Geometry: final body of the model. Coordinates: model frame, mm. A direction names the side the tool comes from. Coordinates: 2 decimals unless noted, no trailing zeros. Order: outer loops, then holes, each group sorted by start corner. A loop starts at its lowest first (then second) coordinate and runs counter-clockwise, first axis right, second up. Notation, with made-up numbers: (32.5, 34.5) -> (63.5, 34.5) arc R21 cw to (63.5, 46.5) -> close; hole circle Ø4 at (2, 67.5). An arc over 180 degrees is marked (long way). Use CSV: the item, a comma, the result in double quotes. Start each with the question number.
from build123d import *

# Parameters (mm, degrees)
SKETCH_R    = 7.65
SKETCH_R_2  = 1.6
PAD_DEPTH   = 5
FILLET_R    = 5
FILLET001_R = 5
FILLET002_R = 5


with BuildPart() as part:
    # Sketch → Pad (new body)
    with BuildSketch(Plane.XY):
        Polygon((66, 12.5), (66, -12.5), (41, -12.5), (37, -8.5), (-37, -8.5), (-41, -12.5), (-66, -12.5), (-66, 12.5), (-41, 12.5), (-37, 8.5), (37, 8.5), (41, 12.5), align=None)
        with Locations((54, 0)):
            Circle(SKETCH_R, mode=Mode.SUBTRACT)
        with Locations((45.5, 8.5)):
            Circle(SKETCH_R_2, mode=Mode.SUBTRACT)
        with Locations((62.5, 8.5)):
            Circle(SKETCH_R_2, mode=Mode.SUBTRACT)
        with Locations((62.5, -8.5)):
            Circle(SKETCH_R_2, mode=Mode.SUBTRACT)
        with Locations((45.5, -8.5)):
            Circle(SKETCH_R_2, mode=Mode.SUBTRACT)
        with Locations((-54, 0)):
            Circle(SKETCH_R, mode=Mode.SUBTRACT)
        with Locations((-45.5, 8.5)):
            Circle(SKETCH_R_2, mode=Mode.SUBTRACT)
        with Locations((-62.5, 8.5)):
            Circle(SKETCH_R_2, mode=Mode.SUBTRACT)
        with Locations((-62.5, -8.5)):
            Circle(SKETCH_R_2, mode=Mode.SUBTRACT)
        with Locations((-45.5, -8.5)):
            Circle(SKETCH_R_2, mode=Mode.SUBTRACT)
        with BuildLine():
            ThreePointArc((-28, 5), (-33, 0), (-28, -5))
            Line((-11.5, -5), (-28, -5))
            ThreePointArc((-11.5, -5), (-6.5, 0), (-11.5, 5))
            Line((-28, 5), (-11.5, 5))
        make_face(mode=Mode.SUBTRACT)
        with BuildLine():
            ThreePointArc((18, -5), (23, 0), (18, 5))
            Line((18, 5), (12, 5))
            ThreePointArc((12, 5), (7, 0), (12, -5))
            Line((18, -5), (12, -5))
        make_face(mode=Mode.SUBTRACT)
    extrude(amount=PAD_DEPTH)

    # Fillet
    fillet_edges = [part.edges().sort_by_distance(p)[0] for p in [
        (66, -12.5, 2.5),
        (66, 12.5, 2.5),
        (-66, -12.5, 2.5),
        (-66, 12.5, 2.5),
    ]]
    fillet(fillet_edges, radius=FILLET_R)

    # Fillet001
    fillet001_edges = [part.edges().sort_by_distance(p)[0] for p in [
        (-41, -12.5, 2.5),
        (-37, -8.5, 2.5),
        (37, -8.5, 2.5),
        (41, -12.5, 2.5),
    ]]
    fillet(fillet001_edges, radius=FILLET001_R)

    # Fillet002
    fillet002_edges = [part.edges().sort_by_distance(p)[0] for p in [
        (41, 12.5, 2.5),
        (37, 8.5, 2.5),
        (-41, 12.5, 2.5),
        (-37, 8.5, 2.5),
    ]]
    fillet(fillet002_edges, radius=FILLET002_R)


solid = part.part
(1) Mould query, pull axis Y, two halves, no side actions, for faces 1 (the face through (-36.82, -8.87, 2.54)), 2 (the face through (23, 0, 2)), 3 (the face through (-36.82, 8.87, 2.54)). Classes: pulls with the +Y half, pulls with the -Y half, needs draft (parallel to the pull), parting line crosses it, or undercut.
(2) Section B-B (x = 54). Return loops of the section in (y, z).
(3) Section C-C (x = -26.5). Return loops of the section in (y, z), then the cut area to 3 significant figures.
(4) Section A-A (y = 0). Return loops of the section in (x, z).
(5) Access query for faces 4 (the face through (-20, -5, 2)), 5 (the face through (36.87, -8.89, 2.54)), 6 (the face through (-41.13, 12.11, 2.54)). Directions: +Z, -Z, +X, -X, +Y, -Y. A direction counts if a zero-diameter tool reaches every point of the face in a straight line with its end or side. Return the directions, or none.
(6) Section D-D (z = 1.8). State how many separate pieces and enclosed holes the cut face has, then the cut area to 3 significant figures.
(7) First-contact query: pin 1 (2 mm diameter, centred on x = 29, z = 4, fed in from -Y); pin 2 (1.5 mm diameter, centred on x = -18, z = 2.5, fed in from +Y). Flat tips, straight axial feed; report the tip coordinate or a pass-through.
(8) Line query: line 1 (Y direction, x = 45.5, z = 4); line 2 (Y direction, x = -62.5, z = 1.65); line 3 (X direction, y = -8, z = 4.7). Output: solid intervals per line, ascending. Write a range as from..to.
Check sheet entries:
1,face 1,"pulls with the -Y half"
1,face 2,"undercut"
1,face 3,"pulls with the +Y half"
2,outline,"(-12.5, 0) -> (-7.65, 0) -> (-7.65, 5) -> (-12.5, 5) -> close; (7.65, 0) -> (12.5, 0) -> (12.5, 5) -> (7.65, 5) -> close"
3,outline,"(-8.5, 0) -> (-5, 0) -> (-5, 5) -> (-8.5, 5) -> close; (5, 0) -> (8.5, 0) -> (8.5, 5) -> (5, 5) -> close"
3,area,"35.0 mm^2"
4,outline,"(-66, 0) -> (-61.65, 0) -> (-61.65, 5) -> (-66, 5) -> close; (-46.35, 0) -> (-33, 0) -> (-33, 5) -> (-46.35, 5) -> close; (-6.5, 0) -> (7, 0) -> (7, 5) -> (-6.5, 5) -> close; (23, 0) -> (46.35, 0) -> (46.35, 5) -> (23, 5) -> close; (61.65, 0) -> (66, 0) -> (66, 5) -> (61.65, 5) -> close"
5,face 4,"+Z, -Z"
5,face 5,"+Z, -Z, -Y"
5,face 6,"+Z, -Z, +Y"
6,separate pieces,"1"
6,enclosed holes,"12"
6,area,"1,840 mm^2"
7,pin 1,"stops at y = -8.5"
7,pin 2,"stops at y = 8.5"
8,line 1,"y = -12.5..-10.1, -6.9..6.9, 10.1..12.5"
8,line 2,"y = -12.27..-10.1, -6.9..6.9, 10.1..12.27"
8,line 3,"x = -65.97..-64.02, -60.98..-47.02, -43.98..43.98, 47.02..60.98, 64.02..65.97"
